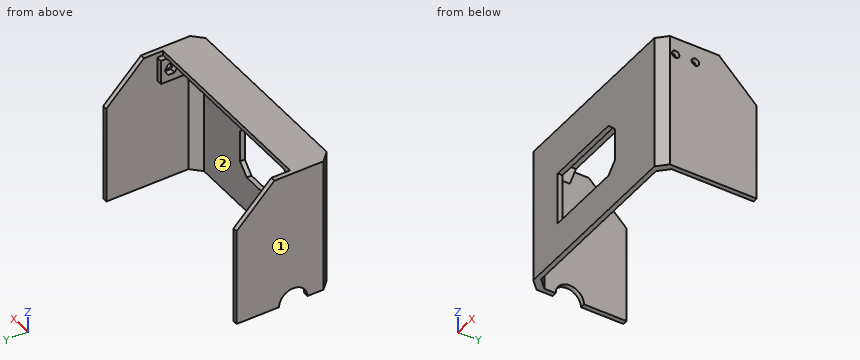
from build123d import *

# Parameters (mm, degrees)
F0_W      = 109
F0_H      = 72
F1_DEPTH  = 51
F2_T      = -2.5
F3_W      = 104
F3_H      = 30
F4_DEPTH  = 2.5
F5_R      = 2
F6_DEPTH  = 2.5
F7_SIZE   = 20
F8_W      = 104
F8_H      = 48.5
F9_DEPTH  = 2.5
F11_DEPTH = 2.5
F14_DEPTH = 3
F15_DEPTH = 2.5
F16_SIZE  = 5
F17_SIZE  = 5


with BuildPart() as f1:
    # F0 (on Front) → F1 (new body)
    with BuildSketch(Plane.XZ):
        with Locations((54.5, 36)):
            Rectangle(F0_W, F0_H)
    extrude(amount=F1_DEPTH)

    # F2
    f2_openings = [f1.faces().sort_by_distance(p)[0] for p in [
        (54.5, 0, 36),
    ]]
    offset(amount=F2_T, openings=f2_openings)

    # F3 (on face) → F4 (cut, through all)
    with BuildSketch(Plane.XY.offset(72)):
        with Locations((54.5, -15)):
            Rectangle(F3_W, F3_H)
    extrude(amount=-F4_DEPTH, mode=Mode.SUBTRACT)

    # F5 (on face) → F6 (cut, through all)
    with BuildSketch(Plane.YZ.offset(109)):
        with Locations((-43, 63)):
            Circle(F5_R)
        with Locations((-32.5, 63)):
            Circle(F5_R)
    extrude(amount=-F6_DEPTH, mode=Mode.SUBTRACT)

    # F7
    f7_edges = [f1.edges().sort_by_distance(p)[0] for p in [
        (107.75, 0, 72),
        (1.25, 0, 72),
    ]]
    chamfer(f7_edges, length=F7_SIZE)

    # F8 (on face) → F9 (cut, through all)
    with BuildSketch(Plane(origin=(0, 0, 0), x_dir=(1, 0, 0), z_dir=(0, 0, -1))):
        with Locations((54.5, 24.25)):
            Rectangle(F8_W, F8_H)
    extrude(amount=-F9_DEPTH, mode=Mode.SUBTRACT)

    # F10 (on face) → F11 (cut, through all)
    with BuildSketch(Plane(origin=(0, 0, 0), x_dir=(0, -1, 0), z_dir=(-1, 0, 0))):
        with BuildLine():
            Line((22.5, 0), (37.5, 0))
            ThreePointArc((37.5, 0), (30, 7.5), (22.5, 0))
        make_face()
    extrude(amount=-F11_DEPTH, mode=Mode.SUBTRACT)

    # F13 (on face) → F14 (join)
    with BuildSketch(Plane(origin=(106.5, 0, 0), x_dir=(0, -1, 0), z_dir=(-1, 0, 0))):
        Polygon((48.5, 56.5), (48.5, 69.5), (30, 69.5), (27, 69.5), (27, 56.5), align=None)
        Polygon((29.0358983849, 63), (30.7679491924, 66), (34.2320508076, 66), (35.9641016151, 63), (34.2320508076, 60), (30.7679491924, 60), align=None, mode=Mode.SUBTRACT)
        Polygon((39.5358983849, 63), (41.2679491924, 66), (44.7320508076, 66), (46.4641016151, 63), (44.7320508076, 60), (41.2679491924, 60), align=None, mode=Mode.SUBTRACT)
    extrude(amount=F14_DEPTH)

    # F12 (on face) → F15 (cut, through all)
    with BuildSketch(Plane.XZ.offset(51)):
        Polygon((66.5, 47), (25, 47), (25, 19), (66.5, 19), (72, 24.5), (72, 41.5), align=None)
    extrude(amount=-F15_DEPTH, mode=Mode.SUBTRACT)

    # F16 (call 1 of 2: OpenCascade refuses the feature's edges together)
    f16_edges = [f1.edges().sort_by_distance(p)[0] for p in [
        (2.5, -48.5, 34.75),
        (2.5, -39.25, 69.5),
        (53, -48.5, 69.5),
    ]]
    chamfer(f16_edges, length=F16_SIZE)

    # F16#2 (call 2 of 2)
    f16_2_edges = [f1.edges().sort_by_distance(p)[0] for p in [
        (106.5, -48.5, 28.25),
    ]]
    chamfer(f16_2_edges, length=F16_SIZE)

    # F17
    f17_edges = [f1.edges().sort_by_distance(p)[0] for p in [
        (0, -51, 36),
        (109, -51, 36),
    ]]
    chamfer(f17_edges, length=F17_SIZE)


solid = f1.part
Part model, mm, in its own coordinate system. Face numbers are marked on the shaded views. A direction names the side the tool comes from. Coordinates: 2 decimals unless noted, no trailing zeros. Write each loop counter-clockwise with the first axis right and the second up, starting at its lowest first coordinate (ties: lowest second). Pieces come first, ordered by that corner, then holes. Notation, with made-up numbers: (-32, 82) - (-5, 82) arc R34 ccw to (-5, 121) - close; hole circle Ø2 at (28, 83). An arc over 180 degrees is marked (long way). Put each result on its own line as item: value.
1. Band-saw the part on C-C (x = 39.5). Write the cut outline in (y, z), then the cut area to 3 significant figures.
Final values:
outline: (-51, 0) - (-48.5, 0) - (-48.5, 19) - (-51, 19) - close; (-51, 47) - (-48.5, 47) - (-48.5, 64.5) - (-43.5, 69.5) - (-30, 69.5) - (-30, 72) - (-51, 72) - close
area: 169 mm²
2. Band-saw the part on D-D (x = 92). Write the cut outline in (y, z).
Final values:
outline: (-51, 0) - (-48.5, 0) - (-48.5, 64.5) - (-43.5, 69.5) - (-30, 69.5) - (-30, 72) - (-51, 72) - close
3. 3-axis set-ups, long thin cutter, end or side, ignore diameter. For the marked faces 1 and 2: which of +Z, -Z, +X, -X, +Y, -Y reach the whole face in a straight line?
Final values:
face 1: +Z, -Z, -X, +Y, -Y
face 2: -Z, +Y
4. Band-saw the part on B-B (z = 32.5). Write the cut outline in (x, y), then the cut area to 4 significant figures.
Final values:
outline: (0, -46) - (5, -51) - (25, -51) - (25, -48.5) - (7.5, -48.5) - (2.5, -43.5) - (2.5, 0) - (0, 0) - close; (72, -51) - (104, -51) - (109, -46) - (109, 0) - (106.5, 0) - (106.5, -43.5) - (101.5, -48.5) - (72, -48.5) - close
area: 397.5 mm²
5. Flat gauge pins, fed straight in: pin 1 Ø3.5 at (x, y) = (104.5, -32.5) entering from -Z; pin 2 Ø2 at (y, z) = (-49.5, 34.5) entering from -X; pin 3 Ø1 at (x, z) = (14.5, 20.5) entering from +Y; pin 4 Ø12 at (x, y) = (36.5, -22) entering from +Z. Where does each tip first touch, or does it go through?
Final values:
pin 1: stops at z = 56.5
pin 2: stops at x = 2.5
pin 3: stops at y = -48.5
pin 4: passes through
6. Probe line 1 along X through (y, z) = (-5, 40); line 2 along Z through (x, y) = (107.95, -32.5); line 3 along Y through (x, z) = (52, 59.5). List the from-to ranges inside material, lowest first. Write a range as [from, to].
Final values:
line 1: x = [0, 2.5], [106.5, 109]
line 2: z = [0, 61], [65, 72]
line 3: y = [-51, -48.5]
7. Band-saw the part on A-A (y = -9). Write the cut outline in (x, z).
Final values:
outline: (0, 0) - (2.5, 0) - (2.5, 61) - (0, 61) - close; (106.5, 0) - (109, 0) - (109, 61) - (106.5, 61) - close
